The model under review builds one solid part; all positions refer to its coordinate system, in mm. A direction names the side the tool comes from. Round coordinates to 2 decimals unless told otherwise and drop trailing zeros. Order: outer loops, then holes, each group sorted by start corner. A loop starts at its lowest first (then second) coordinate and runs counter-clockwise, first axis right, second up.
```python
from build123d import *

# Parameters (mm, degrees)
F1_DEPTH = 90
F3_D     = 3


with BuildPart() as f1:
    # F0 (on Top) → F1 (new body, symmetric)
    with BuildSketch(Plane.XY):
        Polygon((-6.5, 6.5), (-7.5, 7.5), (-7.5, -7.5), (7.5, -7.5), (6.5, -6.5), (-6.5, -6.5), align=None)
        Polygon((7.5, 7.5), (-7.5, 7.5), (-6.5, 6.5), (6.5, 6.5), (6.5, -6.5), (7.5, -7.5), align=None)
    extrude(amount=F1_DEPTH, both=True)

    # F3 (through all)
    with Locations(Plane(origin=(-7.5, 0, 0), x_dir=(0, -1, 0), z_dir=(-1, 0, 0))):
        with Locations((0, 82.5), (0, -82.5)):
            Hole(F3_D / 2)


solid = f1.part
```
(1) For faces 5 (the flat face through (0, -6.5, 1)), 6 (the flat face through (7.5, 0, 1)), list the 3-axis set-ups (+Z, -Z, +X, -X, +Y, -Y) from which the entire face can be reached by the end or side of a thin tool; tool diameter is ignored.
Data:
face 5: +Z, -Z
face 6: +Z, -Z, +X, +Y, -Y
(2) To check wall thickness, follow probe 1 along Z at (x, y) = (7.2, 0); probe 2 along Y at (x, z) = (3, 15.5). State the ranges of each line that lie inside material, in increasing order.
Data:
probe 1: z = -90 to -84, -81 to 81, 84 to 90
probe 2: y = -7.5 to -6.5, 6.5 to 7.5
(3) Consider section A-A (x = 0). Write out the cut boundary in (y, z).
Data:
outline: (-7.5, -90) - (-6.5, -90) - (-6.5, 90) - (-7.5, 90) - close; (6.5, -90) - (7.5, -90) - (7.5, 90) - (6.5, 90) - close
(4) Consider section B-B (z = -30). Write out the cut boundary in (x, y).
Data:
outline: (-7.5, -7.5) - (7.5, -7.5) - (7.5, 7.5) - (-7.5, 7.5) - close; hole (-6.5, -6.5) - (6.5, -6.5) - (6.5, 6.5) - (-6.5, 6.5) - close
(5) Draft analysis for pull direction Z (two halves, no side actions). For faces 1 (the cylindrical face through (-7, 0, 84)), 2 (the flat face through (-7, 0, -90)), 3 (the flat face through (0, -7.5, 1)), 4 (the cylindrical face through (7, 0, 84)), state which applies: pulls with the +Z half, pulls with the -Z half, needs draft (parallel to the pull), parting line crosses it, or undercut.
Data:
face 1: undercut
face 2: pulls with the -Z half
face 3: needs draft
face 4: undercut
(6) Consider section D-D (z = 82.5). Write out the cut boundary in (x, y).
Data:
outline: (-7.5, -7.5) - (7.5, -7.5) - (7.5, -1.5) - (6.5, -1.5) - (6.5, -6.5) - (-6.5, -6.5) - (-6.5, -1.5) - (-7.5, -1.5) - close; (-7.5, 1.5) - (-6.5, 1.5) - (-6.5, 6.5) - (6.5, 6.5) - (6.5, 1.5) - (7.5, 1.5) - (7.5, 7.5) - (-7.5, 7.5) - close
(7) Insertion check: pin 1 (3.5 mm diameter, centred on y = 0, z = -82.5, fed in from +X); pin 2 (1.8 mm diameter, centred on y = 0, z = 82.5, fed in from -X). Each pin has a flat end and moves straight along its axis. Give the tip position at first contact, or say it passes through.
Data:
pin 1: stops at x = 7.5
pin 2: passes through
